```python
from build123d import *

# Parameters (mm, degrees)
BOSS_EXTRUDE1_DEPTH     = 92.5
CUT_EXTRUDE2_DEPTH      = 158.5
CUT_EXTRUDE2_DEPTH_BACK = 158.5
SKETCH3_R               = 1.5
SKETCH4_W               = 40
SKETCH4_H               = 165
BOSS_EXTRUDE2_DEPTH     = 2.5


with BuildPart() as part:
    # Sketch1 → Boss-Extrude1 (new, symmetric)
    with BuildSketch(Plane.XY):
        with BuildLine():
            Line((-40, 55), (-60, 55))
            ThreePointArc((-60, 55), (-115, 0), (-60, -55))
            Line((-60, -55), (-40, -55))
            Line((-40, -55), (-40, -52.5))
            Line((-40, -52.5), (-60, -52.5))
            ThreePointArc((-60, -52.5), (-112.5, 0), (-60, 52.5))
            Line((-60, 52.5), (-40, 52.5))
            Line((-40, 52.5), (-40, 55))
        make_face()
    extrude(amount=BOSS_EXTRUDE1_DEPTH, both=True)

    # Sketch3 → Cut-Extrude2 (cut, two sides: drawn at the far end of the back side and taken through both)
    with BuildSketch(Plane(origin=(0, 0, 0), x_dir=(1, 0, 0), z_dir=(0, 1, 0)).offset(-CUT_EXTRUDE2_DEPTH_BACK)):
        with Locations(Location((-55, 88.75, 0), (0, 0, 270))):
            Circle(SKETCH3_R)
        with Locations((-33, 88.75)):
            Circle(SKETCH3_R)
        with Locations((-11, 88.75)):
            Circle(SKETCH3_R)
        with Locations((-11, -88.75)):
            Circle(SKETCH3_R)
        with Locations((-33, -88.75)):
            Circle(SKETCH3_R)
        with Locations(Location((-55, -88.75, 0), (0, 0, 270))):
            Circle(SKETCH3_R)
    extrude(amount=CUT_EXTRUDE2_DEPTH + CUT_EXTRUDE2_DEPTH_BACK, mode=Mode.SUBTRACT)

    # Sketch4 → Boss-Extrude2 (add)
    with BuildSketch(Plane(origin=(0, 55, 0), x_dir=(1, 0, 0), z_dir=(0, 1, 0))):
        with Locations((-20, 0)):
            Rectangle(SKETCH4_W, SKETCH4_H)
    extrude(amount=-BOSS_EXTRUDE2_DEPTH)


solid = part.part
```
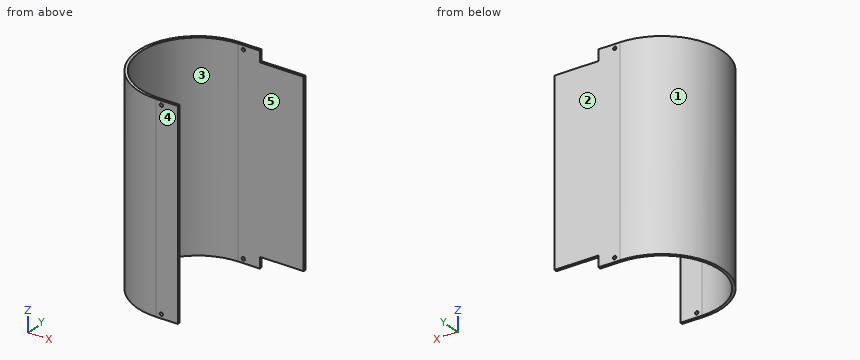
Check sheet for the modelled part. Datum: model origin and axes. Units: mm. Face numbers are marked on the shaded views. A direction names the side the tool comes from. Round coordinates to 2 decimals unless told otherwise and drop trailing zeros. Write each loop counter-clockwise with the first axis right and the second up, starting at its lowest first coordinate (ties: lowest second). Pieces come first, ordered by that corner, then holes. Notation, with made-up numbers: (36, 89) -> (86, 89) arc R10 ccw to (86, 104) -> close; hole circle Ø2 at (10.5, 27.25). An arc over 180 degrees is marked (long way). One line per question, with ' | ' between items. Start each with the question number.
1. Depth check by flat-ended pin: pin 1 (3 mm diameter, centred on y = 35.5, z = 53, fed in from +X); pin 2 (3 mm diameter, centred on y = 53, z = 88, fed in from +X); pin 3 (1.5 mm diameter, centred on y = 20, z = -26, fed in from -X). Enter the tip coordinate at first touch or a pass-through.
2. Sectioned sample at A-A, the plane x = -94. Record the cut outline in (y, z).
3. Scan lines: line 1 along Z through (x, y) = (-55, 53); line 2 along Y through (x, z) = (-46, -30); line 3 along Y through (x, z) = (-31.5, -23). Record each from-to range of solid material in increasing order. Write a range as from..to.
4. Release check for a two-part mould opening along Y. For the marked faces 1, 2 and 3 record: +Y half, -Y half, draft (parallel to the pull), parting line (faces both ways), or undercut.
5. Set-up check for the marked faces 4 and 5: record each of +Z, -Z, +X, -X, +Y, -Y from which the full face is reachable in a straight line by a thin tool's end or side.
6. Sectioned sample at B-B, the plane z = 15. Record the cut outline in (x, y).
7. Sectioned sample at C-C, the plane y = 0. Record the cut outline in (x, z), then the cut area to 4 significant figures.
8. Sectioned sample at D-D, the plane x = -20. Record the cut outline in (y, z), then the cut area to 4 significant figures.
Taken from the geometry:
1) pin 1: stops at x = -97.25 | pin 2: stops at x = -40 | pin 3: stops at x = -111.52
2) outline: (-43.23, -92.5) -> (-40, -92.5) -> (-40, 92.5) -> (-43.23, 92.5) -> close; (40, -92.5) -> (43.23, -92.5) -> (43.23, 92.5) -> (40, 92.5) -> close
3) line 1: z = -92.5..-90.25, -87.25..87.25, 90.25..92.5 | line 2: y = -55..-52.5, 52.5..55 | line 3: y = 52.5..55
4) face 1: parting line | face 2: +Y half | face 3: undercut
5) face 4: +Z, -Z, +X, -X, -Y | face 5: +Z, -Z, +X
6) outline: (-60, -55) -> (-40, -55) -> (-40, -52.5) -> (-60, -52.5) arc R52.5 cw to (-60, 52.5) -> (0, 52.5) -> (0, 55) -> (-60, 55) arc R55 ccw to start
7) outline: (-115, -92.5) -> (-112.5, -92.5) -> (-112.5, 92.5) -> (-115, 92.5) -> close | area: 462.5 mm^2
8) outline: (52.5, -82.5) -> (55, -82.5) -> (55, 82.5) -> (52.5, 82.5) -> close | area: 412.5 mm^2
